from build123d import *

# Parameters (mm, degrees)
ESQUISSE1_R             = 19.05
BOSS_EXTRU_1_DEPTH      = 50.8
ESQUISSE6_W             = 4.1275
ESQUISSE6_H             = 38.1
ENL_V_MAT_EXTRU_1_DEPTH = 38.1
ESQUISSE7_W             = 4.1275
ESQUISSE7_H             = 38.1
ENL_V_MAT_EXTRU_2_DEPTH = 38.1


with BuildPart() as part:
    # Esquisse1 → Boss.-Extru.1 (new body)
    with BuildSketch(Plane.XY):
        Circle(ESQUISSE1_R)
    extrude(amount=BOSS_EXTRU_1_DEPTH)

    # Esquisse6 → Enlèv. mat.-Extru.1 (cut)
    with BuildSketch(Plane(origin=(0, 0, 0), x_dir=(-1, 0, 0), z_dir=(0, 0, -1))):
        with Locations((4.22275, 0)):
            Rectangle(ESQUISSE6_W, ESQUISSE6_H)
    extrude(amount=-ENL_V_MAT_EXTRU_1_DEPTH, mode=Mode.SUBTRACT)

    # Esquisse7 → Enlèv. mat.-Extru.2 (cut)
    with BuildSketch(Plane(origin=(0, 0, 0), x_dir=(-1, 0, 0), z_dir=(0, 0, -1))):
        with Locations((-4.22275, 0)):
            Rectangle(ESQUISSE7_W, ESQUISSE7_H)
        with Locations((-12.66825, 0)):
            Rectangle(ESQUISSE7_W, ESQUISSE7_H)
        with Locations((12.66825, 0)):
            Rectangle(ESQUISSE7_W, ESQUISSE7_H)
    extrude(amount=-ENL_V_MAT_EXTRU_2_DEPTH, mode=Mode.SUBTRACT)


solid = part.part
The model under review builds one solid part; all positions refer to its coordinate system, in mm. A direction names the side the tool comes from. Round coordinates to 2 decimals unless told otherwise and drop trailing zeros. Order: outer loops, then holes, each group sorted by start corner. A loop starts at its lowest first (then second) coordinate and runs counter-clockwise, first axis right, second up. Notation, with made-up numbers: (-28, -27.5) - (18, -27.5) arc R17 ccw to (18, -2.5) - close; hole circle Ø8 at (-25.75, 72). An arc over 180 degrees is marked (long way). Use one line per item in the form item = value.
Q1. Add section C-C on z = 47.5. Give the boundary of the cut face in (x, y), then the cut area to 3 significant figures.
Response values:
outline = circle Ø38.1 at (0, 0)
area = 1,140 mm^2
Q2. Add section A-A on z = 5. Give the boundary of the cut face in (x, y), then the cut area to 3 significant figures.
Response values:
outline = (-14.73, -12.08) - (-14.73, 12.08) arc R19.05 ccw to start; (-10.6, -15.83) arc R19.05 ccw to (-6.29, -17.98) - (-6.29, 17.98) arc R19.05 ccw to (-10.6, 15.83) - close; (-2.16, -18.93) arc R19.05 ccw to (2.16, -18.93) - (2.16, 18.93) arc R19.05 ccw to (-2.16, 18.93) - close; (6.29, -17.98) arc R19.05 ccw to (10.6, -15.83) - (10.6, 15.83) arc R19.05 ccw to (6.29, 17.98) - close; (14.73, -12.08) arc R19.05 ccw to (14.73, 12.08) - close
area = 601 mm^2
Q3. Tool access review of faces 1 (the flat face through (14.732, 0, 19)), 2 (the flat face through (0, 0, 0)): name each direction out of +Z, -Z, +X, -X, +Y, -Y from which nothing blocks a thin tool from reaching the whole face with its end or side.
Response values:
face_1 = -Z, +Y, -Y
face_2 = -Z, +X, -X, +Y, -Y
Q4. Add section D-D on y = 14. Give the boundary of the cut face in (x, z).
Response values:
outline = (-12.92, 38.1) - (-10.6, 38.1) - (-10.6, 0) - (-6.29, 0) - (-6.29, 38.1) - (-2.16, 38.1) - (-2.16, 0) - (2.16, 0) - (2.16, 38.1) - (6.29, 38.1) - (6.29, 0) - (10.6, 0) - (10.6, 38.1) - (12.92, 38.1) - (12.92, 50.8) - (-12.92, 50.8) - close
Q5. Mouldability with a two-part tool opening along X and no side actions: class faces 3 (the flat face through (-14.732, 0, 19)), 4 (the cylindrical face through (17.597, -7.296, 25.044)), 5 (the flat face through (8, 0, 0)) as pulls with the +X half, pulls with the -X half, needs draft (parallel to the pull), parting line crosses it, or undercut.
Response values:
face_3 = undercut
face_4 = parting line crosses it
face_5 = needs draft
Q6. Add section B-B on y = 0. Give the boundary of the cut face in (x, z), then the cut area to 3 significant figures.
Response values:
outline = (-19.05, 0) - (-14.73, 0) - (-14.73, 38.1) - (-10.6, 38.1) - (-10.6, 0) - (-6.29, 0) - (-6.29, 38.1) - (-2.16, 38.1) - (-2.16, 0) - (2.16, 0) - (2.16, 38.1) - (6.29, 38.1) - (6.29, 0) - (10.6, 0) - (10.6, 38.1) - (14.73, 38.1) - (14.73, 0) - (19.05, 0) - (19.05, 50.8) - (-19.05, 50.8) - close
area = 1,310 mm^2
Q7. To check wall thickness, follow line 1 (X direction, y = -0.5, z = 11.5); line 2 (X direction, y = -15.5, z = 3.5); line 3 (X direction, y = 7.5, z = 9). State the ranges of each line that lie inside material, in increasing order.
Response values:
line_1 = -19.04 to -14.73, -10.6 to -6.29, -2.16 to 2.16, 6.29 to 10.6, 14.73 to 19.04
line_2 = -10.6 to -6.29, -2.16 to 2.16, 6.29 to 10.6
line_3 = -17.51 to -14.73, -10.6 to -6.29, -2.16 to 2.16, 6.29 to 10.6, 14.73 to 17.51
Q8. Clearance check with flat-ended pins moving along their axes: P1, Ø8, axis at x = -6, z = 31, coming from the -Y side; P2, Ø8, axis at y = 10.5, z = 15, coming from the -X side; P3, Ø2, axis at x = -10, z = 21.5, coming from the +Y side. State where each tip first meets the part, or that it passes through.
Response values:
P1 = -18.94
P2 = -17.91
P3 = 16.79
